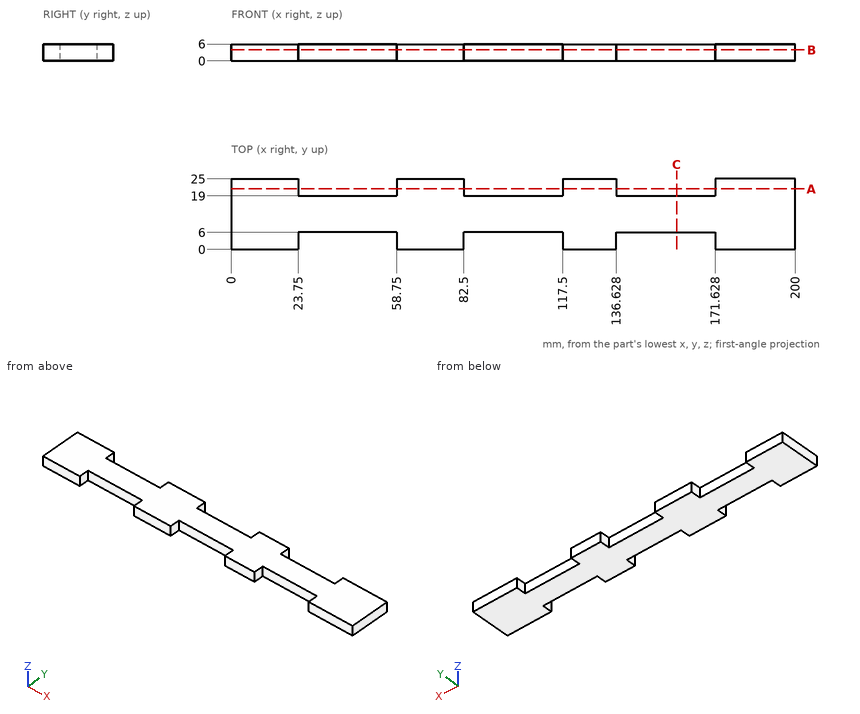
Could you check a few things on this drawing? It's one solid part, dimensions in mm from its lowest x, y, z. Give positions to 0.01 mm unless a question says otherwise; leave off trailing zeros. Loops run counter-clockwise (first coordinate to the right, second up) from the corner with the lowest first, then second, coordinate; pieces in that order, holes last. Notation, with made-up numbers: M -18,66.25 L 35,66.25 A18 cw 35,88.25 Z; hole C 47,58.5 d5. An arc over 180 degrees is marked long. Return JSON: item names as keys, results as strings.
Item 1: Imagine slicing it at C-C on x = 158. List the corners of the cut face in (y, z) for me.
A:
{"outline": "M 6,0 L 19,0 L 19,6 L 6,6 Z"}
Item 2: Please list where these lines run through material, in increasing order: line 1 (X direction, y = 1.75, z = 5.35); line 2 (Y direction, x = 148, z = 1.9).
A:
{"line 1": "x = 0 to 23.75, 58.75 to 82.5, 117.5 to 136.63, 171.63 to 200", "line 2": "y = 6 to 19"}
Item 3: I'm going to push flat-ended pins straight in: pin 1 Ø1.8 at (y, z) = (23.5, 2.5) entering from -X; pin 2 Ø1.8 at (x, z) = (160, 2) entering from -Y; pin 3 Ø1.8 at (x, z) = (46, 3) entering from +Y. Where does each tip first touch, or does it pass through?
A:
{"pin 1": "stops at x = 0", "pin 2": "stops at y = 6", "pin 3": "stops at y = 19"}
Item 4: Imagine slicing it at B-B on z = 3.95. List the corners of the cut face in (x, y) for me.
A:
{"outline": "M 0,0 L 23.75,0 L 23.75,6 L 58.75,6 L 58.75,0 L 82.5,0 L 82.5,6 L 117.5,6 L 117.5,0 L 136.63,0 L 136.63,6 L 171.63,6 L 171.63,0 L 200,0 L 200,25 L 171.63,25 L 171.63,19 L 136.63,19 L 136.63,25 L 117.5,25 L 117.5,19 L 82.5,19 L 82.5,25 L 58.75,25 L 58.75,19 L 23.75,19 L 23.75,25 L 0,25 Z"}
Item 5: Imagine slicing it at A-A on y = 21.5. List the corners of the cut face in (x, z) for me, then the cut area to 3 significant figures.
A:
{"outline": "M 0,0 L 23.75,0 L 23.75,6 L 0,6 Z; M 58.75,0 L 82.5,0 L 82.5,6 L 58.75,6 Z; M 117.5,0 L 136.63,0 L 136.63,6 L 117.5,6 Z; M 171.63,0 L 200,0 L 200,6 L 171.63,6 Z", "area": "570 mm^2"}
